Can you work these out from the drawing? Everything is in mm from the part's minimum corner. A direction names the side the tool comes from. Round coordinates to 2 decimals unless told otherwise and drop trailing zeros. Write each loop counter-clockwise with the first axis right and the second up, starting at its lowest first coordinate (ties: lowest second). Pieces come first, ordered by that corner, then holes. Notation, with made-up numbers: (21.5, 23) - (71.5, 23) arc R38 ccw to (71.5, 62) - close; hole circle Ø5 at (22, -12.75). An arc over 180 degrees is marked (long way). One line per item, written item: value. Start each with the question number.
(1) Thinking about a two-plate mould opening in Y: for the marked faces 3, 4, 5 and 6, which applies, +Y half, -Y half, draft (parallel to the pull), parting line (faces both ways), or undercut?
(2) On a 3-axis mill with a long thin cutter (end or side, diameter ignored), from which of +Z, -Z, +X, -X, +Y, -Y can I reach the whole of each face in a straight line? I mean the marked faces 1 and 2. Say none if no direction works.
(3) If I drill on L1, parallel to Y at x = 11.25, z = 16 (1 decimal); L2, parallel to Z at x = 18.25, y = 5.5; L3, parallel to X at y = 11.25, z = 8.5 (1 decimal), over which ranges is the centre line in solid material (lowest first)? Write a range as from..to.
(4) I'm going to push flat-ended pins straight in: pin 1 Ø3 at (y, z) = (6.5, 15) entering from -X; pin 2 Ø6 at (y, z) = (13.5, 13) entering from +X; pin 3 Ø2 at (y, z) = (11, 14) entering from -X. Where does each tip first touch, or does it pass through?
(5) I want a section at B-B on x = 16. List the corners of the cut face in (y, z) for me.
(6) I want a section at A-A on z = 2.5. List the corners of the cut face in (x, y) for me (1 decimal), plus the area to 3 significant figures.
(7) I want a section at C-C on y = 19. List the corners of the cut face in (x, z) for me (1 decimal).
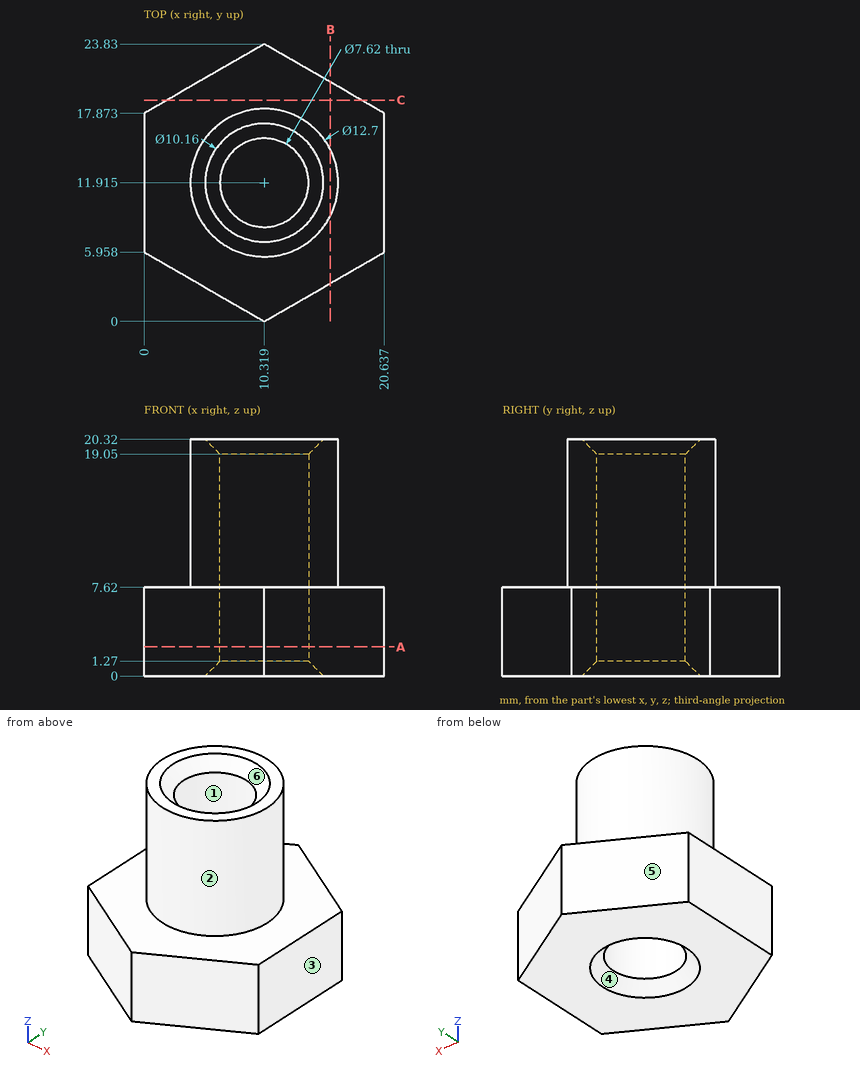
Established:
1. face 3: draft
1. face 4: undercut
1. face 5: +Y half
1. face 6: undercut
2. face 1: +Z, -Z
2. face 2: +Z
3. L1: 5.6..8.2, 15.6..18.2
3. L2: 0..7.62
3. L3: 4..6.6, 14.1..16.6
4. pin 1: x = 5.32
4. pin 2: x = 16.67
4. pin 3: x = 3.97
5. outline: (3.28, 0) - (20.55, 0) - (20.55, 7.62) - (14.75, 7.62) - (14.75, 20.32) - (9.08, 20.32) - (9.08, 7.62) - (3.28, 7.62) - close
6. outline: (0, 6) - (10.3, 0) - (20.6, 6) - (20.6, 17.9) - (10.3, 23.8) - (0, 17.9) - close; hole circle Ø7.6 at (10.3, 11.9)
6. area: 323 mm2
7. outline: (2, 0) - (18.7, 0) - (18.7, 7.6) - (2, 7.6) - close
